Geometry check sheet. Reference: the model listing, model coordinates, mm. Face numbers are marked on the shaded views. A direction names the side the tool comes from. Give positions to 0.01 mm unless a question says otherwise; leave off trailing zeros. Write each loop counter-clockwise with the first axis right and the second up, starting at its lowest first coordinate (ties: lowest second). Pieces come first, ordered by that corner, then holes. Notation, with made-up numbers: (77, 15) - (86, 15) arc R10 cw to (86, 31) - close; hole circle Ø1 at (-24, 16). An arc over 180 degrees is marked (long way). Write item = value, one per line. Start each with the question number.
(1) Thickness scan on L1, parallel to Z at x = 0, y = -0.15; L2, parallel to Y at x = 0.5, z = 33; L3, parallel to Y at x = 5, z = 36 (3 decimals). Record the ranges inside material, lowest first.
(2) Section check B-B, the plane x = 17. Enter the section's corners in (y, z), plus the area to 3 significant figures.
(3) Section check A-A, the plane z = 12. Enter the section's corners in (x, y), plus the area to 3 significant figures.
(4) Section check C-C, the plane z = 29. Enter the section's corners in (x, y).
(5) Depth check by flat-ended pin: pin 1 Ø1.2 at (x, y) = (33, 2.5) entering from -Z; pin 2 Ø22 at (x, z) = (0, 41.34) entering from +Y; pin 3 Ø18 at (x, z) = (0.5, 38) entering from -Y. Enter the tip coordinate at first touch or a pass-through.
(6) Access from +Z, -Z, +X, -X, +Y, -Y to the whole of each face (thin tool, end or side, straight path). Record for the marked faces 1, 2 and 3.
```python
from build123d import *

# Parameters (mm, degrees)
F0_R     = 32.3708711279
F1_DEPTH = 12.7
F2_R     = 27.3986132433
F3_DEPTH = 12.827
F5_DEPTH = 25.4
F6_R     = 1.27
F8_R     = 8.2490124286
F8_R_2   = 6.9276952265
F9_DEPTH = 0.635


# Not quite as in the source:
# - two fillets or chamfers of one size are made in one step


with BuildPart() as f1:
    # F0 (on Front) → F1 (new body, symmetric)
    with BuildSketch(Plane.XZ):
        Circle(F0_R)
    extrude(amount=F1_DEPTH, both=True)

    # F2 (on Front) → F3 (join, symmetric)
    with BuildSketch(Plane.XZ):
        Circle(F2_R)
    extrude(amount=F3_DEPTH, both=True)

    # F4 (on face) → F5 (join)
    with BuildSketch(Plane.XZ.offset(12.7)):
        with BuildLine():
            ThreePointArc((-24.0273053052, 21.6924387138), (-22.8896624875, 22.8896624875), (-21.6924387138, 24.0273053052))
            Line((-21.6924387138, 24.0273053052), (-22.3403787647, 24.6752453562))
            Line((-22.3403787647, 24.6752453562), (-23.5078120604, 23.5078120604))
            Line((-23.5078120604, 23.5078120604), (-24.6752453562, 22.3403787647))
            Line((-24.6752453562, 22.3403787647), (-24.0273053052, 21.6924387138))
        make_face()
        with BuildLine():
            Line((24.6752453562, 22.3403787647), (23.5078120604, 23.5078120604))
            Line((23.5078120604, 23.5078120604), (22.3403787647, 24.6752453562))
            Line((22.3403787647, 24.6752453562), (21.6924387138, 24.0273053052))
            ThreePointArc((21.6924387138, 24.0273053052), (22.8896624875, 22.8896624875), (24.0273053052, 21.6924387138))
            Line((24.0273053052, 21.6924387138), (24.6752453562, 22.3403787647))
        make_face()
        with BuildLine():
            Line((24.6752453562, -22.3403787647), (24.0273053052, -21.6924387138))
            ThreePointArc((24.0273053052, -21.6924387138), (22.8896624875, -22.8896624875), (21.6924387138, -24.0273053052))
            Line((21.6924387138, -24.0273053052), (22.3403787647, -24.6752453562))
            Line((22.3403787647, -24.6752453562), (23.5078120604, -23.5078120604))
            Line((23.5078120604, -23.5078120604), (24.6752453562, -22.3403787647))
        make_face()
        with BuildLine():
            ThreePointArc((-21.6924387138, -24.0273053052), (-22.8896624875, -22.8896624875), (-24.0273053052, -21.6924387138))
            Line((-24.0273053052, -21.6924387138), (-24.6752453562, -22.3403787647))
            Line((-24.6752453562, -22.3403787647), (-23.5078120604, -23.5078120604))
            Line((-23.5078120604, -23.5078120604), (-22.3403787647, -24.6752453562))
            Line((-22.3403787647, -24.6752453562), (-21.6924387138, -24.0273053052))
        make_face()
        with BuildLine():
            Line((1.651, -33.4515422583), (1.651, -32.3287410299))
            ThreePointArc((1.651, -32.3287410299), (0, -32.3708711279), (-1.651, -32.3287410299))
            Line((-1.651, -32.3287410299), (-1.651, -33.4515422583))
            Line((-1.651, -33.4515422583), (0, -33.4515422583))
            Line((0, -33.4515422583), (1.651, -33.4515422583))
        make_face()
        with BuildLine():
            ThreePointArc((-32.3287410299, -1.651), (-32.3708711279, 0), (-32.3287410299, 1.651))
            Line((-32.3287410299, 1.651), (-33.4515480299, 1.651))
            Line((-33.4515480299, 1.651), (-33.4515480299, 0))
            Line((-33.4515480299, 0), (-33.4515480299, -1.651))
            Line((-33.4515480299, -1.651), (-32.3287410299, -1.651))
        make_face()
        with BuildLine():
            Line((33.4515480299, 1.651), (32.3287410299, 1.651))
            ThreePointArc((32.3287410299, 1.651), (32.3603368894, 0.8257687245), (32.3708711279, 0))
            ThreePointArc((32.3708711279, 0), (32.3603368894, -0.8257687245), (32.3287410299, -1.651))
            Line((32.3287410299, -1.651), (33.4515480299, -1.651))
            Line((33.4515480299, -1.651), (33.4515480299, 0))
            Line((33.4515480299, 0), (33.4515480299, 1.651))
        make_face()
        with BuildLine():
            ThreePointArc((-1.651, 32.3287410299), (0, 32.3708711279), (1.651, 32.3287410299))
            Line((1.651, 32.3287410299), (1.651, 33.4515422583))
            Line((1.651, 33.4515422583), (0, 33.4515422583))
            Line((0, 33.4515422583), (-1.651, 33.4515422583))
            Line((-1.651, 33.4515422583), (-1.651, 32.3287410299))
        make_face()
    extrude(amount=-F5_DEPTH)

    # F6
    f6_edges = [f1.edges().sort_by_distance(p)[0] for p in [
        (24.351275, 12.7, -22.016409),
        (22.016409, 12.7, -24.351275),
        (24.351275, -12.7, -22.016409),
        (22.016409, -12.7, -24.351275),
        (24.351275, -12.7, 22.016409),
        (22.016409, -12.7, 24.351275),
        (22.016409, 12.7, 24.351275),
        (24.351275, 12.7, 22.016409),
        (-22.016409, 12.7, 24.351275),
        (-24.351275, 12.7, 22.016409),
        (-24.351275, 12.7, -22.016409),
        (-22.016409, 12.7, -24.351275),
        (-22.016409, -12.7, -24.351275),
        (-24.351275, -12.7, -22.016409),
        (-24.351275, -12.7, 22.016409),
        (-22.016409, -12.7, 24.351275),
        (32.890145, -12.7, 1.651),
        (32.890145, 12.7, 1.651),
        (1.651, -12.7, 32.890142),
        (-1.651, -12.7, 32.890142),
        (-32.890145, -12.7, 1.651),
        (-32.890145, -12.7, -1.651),
        (-1.651, -12.7, -32.890142),
        (1.651, -12.7, -32.890142),
        (32.890145, -12.7, -1.651),
        (1.651, 12.7, 32.890142),
        (-1.651, 12.7, 32.890142),
        (-32.890145, 12.7, 1.651),
        (-32.890145, 12.7, -1.651),
        (-1.651, 12.7, -32.890142),
        (1.651, 12.7, -32.890142),
        (32.890145, 12.7, -1.651),
    ]]
    fillet(f6_edges, radius=F6_R)

    # F8 (on Front) → F9 (join, symmetric)
    with BuildSketch(Plane.XZ):
        with Locations((0, 41.3398481905)):
            Circle(F8_R)
        with Locations((0, 41.3398481905)):
            Circle(F8_R_2, mode=Mode.SUBTRACT)
    extrude(amount=F9_DEPTH, both=True)


solid = f1.part
```
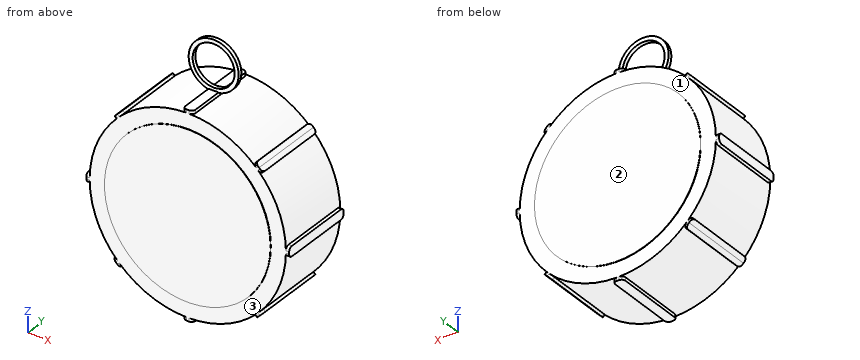
Model answer:
q1.L1 = -33.45 to 34.41, 48.27 to 49.59
q1.L2 = -12.69 to 12.69
q1.L3 = -0.635 to 0.635
q2.outline = (-12.83, -21.49) - (-12.7, -21.49) - (-12.7, -27.55) - (12.7, -27.55) - (12.7, -21.49) - (12.83, -21.49) - (12.83, 21.49) - (12.7, 21.49) - (12.7, 27.55) - (-12.7, 27.55) - (-12.7, 21.49) - (-12.83, 21.49) - close
q2.area = 1,410 mm²
q3.outline = (-30.06, -12.7) - (-24.63, -12.7) - (-24.63, -12.83) - (24.63, -12.83) - (24.63, -12.7) - (30.06, -12.7) - (30.06, 12.7) - (24.63, 12.7) - (24.63, 12.83) - (-24.63, 12.83) - (-24.63, 12.7) - (-30.06, 12.7) - close
q3.area = 1,540 mm²
q4.outline = (-14.38, -12.7) - (14.38, -12.7) - (14.38, 12.7) - (-14.38, 12.7) - close
q5.pin_1 = -1.65
q5.pin_2 = 12.7
q5.pin_3 = -12.7
q6.face_1 = +Y
q6.face_2 = +Z, -Z, +X, -X, +Y
q6.face_3 = -Y
